```python
from build123d import *

# Parameters (mm, degrees)
SKETCH_1_R          = 6.65
EXTRUDE_1_DEPTH     = 1.25
EXTRUDE_2_DEPTH     = 7
SKETCH_3_R          = 1.1
CUT_EXTRUDE_1_DEPTH = 5
CHAMFER_1_SIZE      = 0.7


with BuildPart() as part:
    # Эскиз1 → Бобышка-Вытянуть1 (new, symmetric)
    with BuildSketch(Plane(origin=(0, 0, 0), x_dir=(0, 0, -1), z_dir=(1, 0, 0))):
        with BuildLine():
            Line((-31.25, 0), (-10, 0))
            ThreePointArc((-10, 0), (-2.588190451, -9.659258263), (8.660254038, -5))
            Line((8.660254038, -5), (76.721847542, -5))
            ThreePointArc((76.721847542, -5), (75.425886146, -4.389181279), (74.09117429, -3.868451302))
            ThreePointArc((74.09117429, -3.868451302), (74.147561595, -2.912548148), (74.149130868, -1.954984622))
            ThreePointArc((74.149130868, -1.954984622), (75.638846987, -1.51744657), (77.087831178, -0.959648686))
            ThreePointArc((77.087831178, -0.959648686), (77.109856091, -0.006099484), (77.083941958, 0.947351948))
            ThreePointArc((77.083941958, 0.947351948), (75.643750299, 1.505844774), (74.166291118, 1.956600379))
            ThreePointArc((74.166291118, 1.956600379), (74.147505302, 2.913980899), (74.073940169, 3.8687157))
            ThreePointArc((74.073940169, 3.8687157), (75.433826566, 4.383081961), (76.750365892, 5))
            Line((76.750365892, 5), (8.660254038, 5))
            ThreePointArc((8.660254038, 5), (5, 8.660254038), (0, 10))
            Line((0, 10), (-34.75, 10))
            Line((-34.75, 10), (-34.75, 5))
            Line((-34.75, 5), (-35.25, 5))
            Line((-35.25, 5), (-35.25, 4))
            ThreePointArc((-35.25, 4), (-34.078427125, 1.171572875), (-31.25, 0))
        make_face()
        Circle(SKETCH_1_R, mode=Mode.SUBTRACT)
    extrude(amount=EXTRUDE_1_DEPTH, both=True)

    # Эскиз1<5> → Бобышка-Вытянуть2 (add)
    with BuildSketch(Plane(origin=(0, 0, 0), x_dir=(0, 0, -1), z_dir=(1, 0, 0))):
        with BuildLine():
            Line((73.559260736, 9.685830974), (74.227172899, 10))
            Line((74.227172899, 10), (80.32185029, 10))
            ThreePointArc((80.32185029, 10), (80.927765714, -1.515378033), (79.891173693, -13))
            Line((79.891173693, -13), (75.988629927, -13.007027449))
            ThreePointArc((75.988629927, -13.007027449), (76.159551637, -12.068663477), (76.283109214, -11.12289675))
            ThreePointArc((76.283109214, -11.12289675), (74.948016231, -10.345984286), (73.559260736, -9.669652694))
            ThreePointArc((73.559260736, -9.669652694), (73.690473514, -8.721120367), (73.767167518, -7.766631814))
            ThreePointArc((73.767167518, -7.766631814), (75.28662018, -7.447324325), (76.774901953, -7.004931935))
            ThreePointArc((76.774901953, -7.004931935), (76.871673579, -6.056050262), (76.920646267, -5.103504803))
            ThreePointArc((76.920646267, -5.103504803), (75.528713081, -4.433737489), (74.09117429, -3.868451302))
            ThreePointArc((74.09117429, -3.868451302), (74.147561595, -2.912548148), (74.149130868, -1.954984622))
            ThreePointArc((74.149130868, -1.954984622), (75.638846987, -1.51744657), (77.087831178, -0.959648686))
            ThreePointArc((77.087831178, -0.959648686), (77.109856091, -0.006099484), (77.083941958, 0.947351948))
            ThreePointArc((77.083941958, 0.947351948), (75.643750299, 1.505844774), (74.166291118, 1.956600379))
            ThreePointArc((74.166291118, 1.956600379), (74.147505302, 2.913980899), (74.073940169, 3.8687157))
            ThreePointArc((74.073940169, 3.8687157), (75.524735151, 4.421786748), (76.925488289, 5.091551117))
            ThreePointArc((76.925488289, 5.091551117), (76.872630699, 6.043888899), (76.771989513, 6.992367959))
            ThreePointArc((76.771989513, 6.992367959), (75.292418643, 7.436143003), (73.784148097, 7.769588967))
            ThreePointArc((73.784148097, 7.769588967), (73.691130431, 8.729989779), (73.559260736, 9.685830974))
        make_face()
    extrude(amount=-EXTRUDE_2_DEPTH)

    # Эскиз3 → Вырез-Вытянуть1 (cut)
    with BuildSketch(Plane(origin=(0, 10, 0), x_dir=(1, 0, 0), z_dir=(0, 1, 0))):
        with Locations((0, -35)):
            Circle(SKETCH_3_R)
    extrude(amount=-CUT_EXTRUDE_1_DEPTH, mode=Mode.SUBTRACT)

    # Фаска1
    chamfer_1_edges = [part.edges().sort_by_distance(p)[0] for p in [
        (-1.25, 0, 6.65),
    ]]
    chamfer(chamfer_1_edges, length=CHAMFER_1_SIZE)


solid = part.part
```
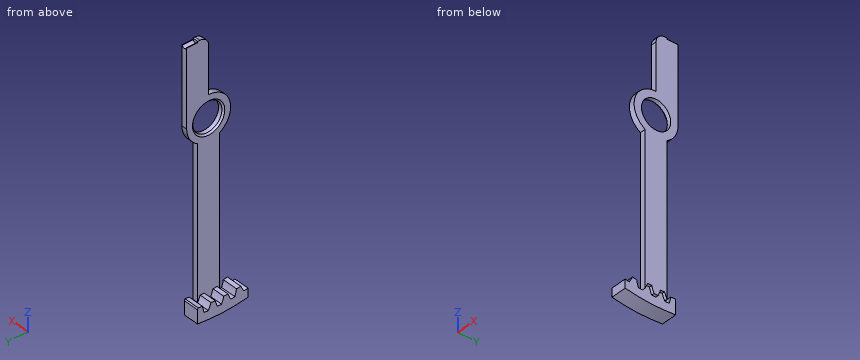
The model under review builds one solid part; all positions refer to its coordinate system, in mm. Coordinates: 2 decimals unless noted, no trailing zeros. Write each loop counter-clockwise with the first axis right and the second up, starting at its lowest first coordinate (ties: lowest second). Pieces come first, ordered by that corner, then holes.
1) We need section B-B on z = 21. State the section outline as (x, y) points, then the cut area to 3 significant figures.
2) To check wall thickness, follow probe 1 along Z at (x, y) = (0.75, -0.5); probe 2 along X at (y, z) = (8.5, 26); probe 3 along X at (y, z) = (-7, -1). State the ranges of each line that lie inside material, in increasing order.
3) We need section A-A on x = -5. State the section outline as (y, z) points.
4) Clearance check with flat-ended pins moving along their axes: pin 1 Ø4 at (x, y) = (-2.5, -2.5) entering from +Z; pin 2 Ø2 at (x, z) = (-0.5, -41) entering from -Y; pin 3 Ø10 at (y, z) = (1.5, -47.5) entering from -X. State where each tip first meets the part, or that it passes through.
Answer list:
1. outline: (-1.25, 0) - (1.25, 0) - (1.25, 10) - (-1.25, 10) - close
1. area: 25.0 mm2
2. probe 1: z = -77.1 to -6.63, 6.63 to 9.99
2. probe 2: x = -1.25 to 1.25
2. probe 3: x = -0.97 to 1.25
3. outline: (-13.01, -75.99) - (-13, -79.89) arc R80.94 ccw to (10, -80.32) - (10, -74.23) - (9.69, -73.56) arc R23.8 cw to (7.77, -73.78) arc R20.93 cw to (6.99, -76.77) arc R18.98 cw to (5.09, -76.93) arc R18.99 cw to (3.87, -74.07) arc R16.72 cw to (1.96, -74.17) arc R20.93 cw to (0.95, -77.08) arc R18.98 cw to (-0.96, -77.09) arc R18.99 cw to (-1.95, -74.15) arc R16.72 cw to (-3.87, -74.09) arc R20.93 cw to (-5.1, -76.92) arc R18.98 cw to (-7, -76.77) arc R18.99 cw to (-7.77, -73.77) arc R16.72 cw to (-9.67, -73.56) arc R20.93 cw to (-11.12, -76.28) arc R18.98 cw to start
4. pin 1: stops at z = 9.96
4. pin 2: stops at y = -5
4. pin 3: stops at x = -1.25
